from build123d import *

# Parameters (mm, degrees)
SKETCH1_R           = 10
SKETCH1_R_2         = 6
BOSS_EXTRUDE1_DEPTH = 12.5
BOSS_EXTRUDE2_DEPTH = 2.5
SKETCH2_3_R         = 2.5
BOSS_EXTRUDE3_DEPTH = 8
SKETCH3_W           = 13
SKETCH3_H           = 8
CUT_EXTRUDE1_DEPTH  = 65.290356975
BOSS_EXTRUDE4_DEPTH = 2.5
SKETCH4_5_R         = 7.5
SKETCH4_5_R_2       = 4
BOSS_EXTRUDE5_DEPTH = 5


with BuildPart() as part:
    # Sketch1 → Boss-Extrude1 (new, symmetric)
    with BuildSketch(Plane.XY):
        Circle(SKETCH1_R)
        Circle(SKETCH1_R_2, mode=Mode.SUBTRACT)
    extrude(amount=BOSS_EXTRUDE1_DEPTH, both=True)

    # Sketch2 → Boss-Extrude2 (add, symmetric)
    with BuildSketch(Plane.XY):
        with BuildLine():
            ThreePointArc((-0.936363066, 9.956064695), (-10, 0), (-0.936363066, -9.956064695))
            Line((-0.936363066, -9.956064695), (-43, -6))
            Line((-43, -6), (-43, 6))
            Line((-43, 6), (-0.936363066, 9.956064695))
        make_face()
    extrude(amount=BOSS_EXTRUDE2_DEPTH, both=True)

    # Sketch2_3 → Boss-Extrude3 (add, symmetric)
    with BuildSketch(Plane.XY):
        with BuildLine():
            Line((-55, 6), (-43, 6))
            Line((-43, 6), (-43, -6))
            Line((-43, -6), (-55, -6))
            ThreePointArc((-55, -6), (-61, 0), (-55, 6))
        make_face()
        with Locations((-55, 0)):
            Circle(SKETCH2_3_R, mode=Mode.SUBTRACT)
    extrude(amount=BOSS_EXTRUDE3_DEPTH, both=True)

    # Sketch3 → Cut-Extrude1 (cut, through all)
    with BuildSketch(Plane(origin=(0, 6, 0), x_dir=(1, 0, 0), z_dir=(0, 1, 0))):
        with Locations((-54.5, 0)):
            Rectangle(SKETCH3_W, SKETCH3_H)
    extrude(amount=-CUT_EXTRUDE1_DEPTH, mode=Mode.SUBTRACT)

    # Sketch4 → Boss-Extrude4 (add, symmetric)
    with BuildSketch(Plane(origin=(0, 0, 0), x_dir=(0.7071067811865512, 0.7071067811865438, 0), z_dir=(-0.7071067811865438, 0.7071067811865512, 0))):
        with BuildLine():
            Line((39, 7.5), (8.997395084, 7.5))
            Line((8.997395084, 7.5), (8.997395084, -7.5))
            Line((8.997395084, -7.5), (39, -7.5))
            ThreePointArc((39, -7.5), (31.5, 0), (39, 7.5))
        make_face()
    extrude(amount=BOSS_EXTRUDE4_DEPTH, both=True)

    # Sketch4_5 → Boss-Extrude5 (add, symmetric)
    with BuildSketch(Plane(origin=(0, 0, 0), x_dir=(0.7071067811865512, 0.7071067811865438, 0), z_dir=(-0.7071067811865438, 0.7071067811865512, 0))):
        with Locations(Location((39, 0, 0), (0, 0, 180))):
            Circle(SKETCH4_5_R)
        with Locations(Location((39, 0, 0), (0, 0, 180))):
            Circle(SKETCH4_5_R_2, mode=Mode.SUBTRACT)
    extrude(amount=BOSS_EXTRUDE5_DEPTH, both=True)


solid = part.part
Can you work these out from the model? Positions are in its coordinate system, mm. A direction names the side the tool comes from. Give positions to 0.01 mm unless a question says otherwise; leave off trailing zeros. Loops run counter-clockwise (first coordinate to the right, second up) from the corner with the lowest first, then second, coordinate; pieces in that order, holes last. Notation, with made-up numbers: (-25.5, 62) -> (28.5, 62) arc R22 cw to (28.5, 80) -> close; hole circle Ø3 at (83, 58.5). An arc over 180 degrees is marked (long way). Return JSON: item names as keys, results as strings.
Q1. We'd pull the mould along Z, two halves only. Please class faces 1 (the face through (32.83, 32.92, 0.33)), 2 (the face through (-48, 0, 0)), 3 (the face through (-6, 0, 0)): released by +Z, released by -Z, zero draft, split by the parting line, or undercut.
Checks:
{"face 1": "split by the parting line", "face 2": "undercut", "face 3": "zero draft"}
Q2. I want a section at B-B, the plane y = 0. List the corners of the cut face in (x, z) for me, then the cut area to 3 significant figures.
Checks:
{"outline": "(-61, -8) -> (-57.5, -8) -> (-57.5, -4) -> (-61, -4) -> close; (-61, 4) -> (-57.5, 4) -> (-57.5, 8) -> (-61, 8) -> close; (-52.5, -8) -> (-43, -8) -> (-43, -2.5) -> (-10, -2.5) -> (-10, -12.5) -> (-6, -12.5) -> (-6, 12.5) -> (-10, 12.5) -> (-10, 2.5) -> (-43, 2.5) -> (-43, 8) -> (-52.5, 8) -> (-52.5, 4) -> (-48, 4) -> (-48, -4) -> (-52.5, -4) -> close; (6, -12.5) -> (10, -12.5) -> (10, 12.5) -> (6, 12.5) -> close", "area": "509 mm2"}
Q3. For pin 1 Ø3 at (y, z) = (0, 4.5) entering from +X; pin 2 Ø6 at (x, y) = (-48.5, 0.5) entering from -Z; pin 3 Ø1.5 at (x, z) = (-27, -4) entering from +Y; pin 4 Ø16 at (x, y) = (-30.5, -5) entering from -Z, each with a flat end and sliding along its axis, tell me the tip position at first contact or that it passes through.
Checks:
{"pin 1": "stops at x = 10", "pin 2": "stops at z = -8", "pin 3": "passes through", "pin 4": "stops at z = -2.5"}
Q4. I want a section at D-D, the plane z = 10.25. List the corners of the cut face in (x, y) for me.
Checks:
{"outline": "circle Ø20 at (0, 0); hole circle Ø12 at (0, 0)"}
Q5. On a 3-axis mill with a long thin cutter (end or side, diameter ignored), from which of +Z, -Z, +X, -X, +Y, -Y can I reach the whole of each face in a straight line? I mean faces 4 (the face through (-22.26, 7.95, 0.04)), 5 (the face through (-43, 0, -5)), 6 (the face through (-52, 0, 4)), 7 (the face through (-52, 0, -8)). Say none if no direction works.
Checks:
{"face 4": "+Z, -Z, -X, +Y", "face 5": "-Z, +Y, -Y", "face 6": "-X, +Y, -Y", "face 7": "-Z, -X, +Y, -Y"}
Q6. I need wall thicknesses on probe 1 along Y at (x, z) = (-55, -7.05); probe 2 along X at (y, z) = (1, -3.75); probe 3 along Z at (x, y) = (-19.5, -7). Which ranges of each line are inside material? Lowest first, please.
Checks:
{"probe 1": "y = -6 to -2.5, 2.5 to 6", "probe 2": "x = -48 to -43, -9.95 to -5.92, 5.92 to 9.95", "probe 3": "z = -2.5 to 2.5"}
Q7. I want a section at A-A, the plane x = 0. List the corners of the cut face in (y, z) for me, then the cut area to 3 significant figures.
Checks:
{"outline": "(-10, -12.5) -> (-6, -12.5) -> (-6, 12.5) -> (-10, 12.5) -> close; (6, -12.5) -> (10, -12.5) -> (10, 12.5) -> (6, 12.5) -> close", "area": "200 mm2"}
Q8. I want a section at C-C, the plane z = -1.25. List the corners of the cut face in (x, y) for me, then the cut area to 3 significant figures.
Checks:
{"outline": "(-48, -6) -> (-43, -6) -> (-0.94, -9.96) arc R10 ccw to (8.61, 5.08) -> (24.12, 20.58) -> (25.88, 18.81) -> (28.43, 21.35) -> (21.35, 28.43) -> (18.81, 25.88) -> (20.58, 24.12) -> (5.08, 8.61) arc R10 ccw to (-0.94, 9.96) -> (-43, 6) -> (-48, 6) -> close; (26.73, 33.8) -> (33.8, 26.73) -> (36.34, 29.27) -> (29.27, 36.34) -> close; hole circle Ø12 at (0, 0)", "area": "974 mm2"}
